```python
from build123d import *

# Parameters (mm, degrees)
BODY_DEPTH                                = 6.75
FILLET1_R                                 = 2.5
F_9_64_0_14063_DIAMETER_HOLE1_D           = 3.572002
F_9_64_0_14063_DIAMETER_HOLE1_DEPTH       = 7
F_9_64_0_14063_DIAMETER_HOLE1_CSINK_D     = 4.842002
F_9_64_0_14063_DIAMETER_HOLE1_CSINK_ANGLE = 45
F_9_64_0_14063_DIAMETER_HOLE1_TIP         = 1.073137666
MOUNT_PEG_DEPTH                           = 3
PEG_CHAMFER_SIZE                          = 0.5


with BuildPart() as part:
    # Sketch1 → body (new body)
    with BuildSketch(Plane.XY):
        with BuildLine():
            Line((6, -23.237900077), (6, -12.760161762))
            Line((6, -12.760161762), (10, -8.760161762))
            Line((10, -8.760161762), (15, -8.760161762))
            Line((15, -8.760161762), (15, -18.734993995))
            ThreePointArc((15, -18.734993995), (10.738670346, -21.463479662), (6, -23.237900077))
        make_face()
    extrude(amount=BODY_DEPTH)

    # Fillet1
    fillet1_edges = [part.edges().sort_by_distance(p)[0] for p in [
        (6, -23.237900077, 3.375),
        (6, -12.760161762, 3.375),
        (10, -8.760161762, 3.375),
        (15, -8.760161762, 3.375),
        (15, -18.734993995, 3.375),
    ]]
    fillet(fillet1_edges, radius=FILLET1_R)

    # 9/64 (0.14063) Diameter Hole1
    with Locations(Plane.ZY.offset(-6)):
        with Locations((4, -17.060161762)):
            CounterSinkHole(F_9_64_0_14063_DIAMETER_HOLE1_D / 2, F_9_64_0_14063_DIAMETER_HOLE1_CSINK_D / 2, depth=F_9_64_0_14063_DIAMETER_HOLE1_DEPTH, counter_sink_angle=F_9_64_0_14063_DIAMETER_HOLE1_CSINK_ANGLE)
            with Locations((0, 0, -(F_9_64_0_14063_DIAMETER_HOLE1_DEPTH + F_9_64_0_14063_DIAMETER_HOLE1_TIP / 2))):  # 118° drill point
                Cone(0, F_9_64_0_14063_DIAMETER_HOLE1_D / 2, F_9_64_0_14063_DIAMETER_HOLE1_TIP, mode=Mode.SUBTRACT)

    # Sketch4 → mount peg (add)
    with BuildSketch(Plane(origin=(0, 0, 0), x_dir=(-1, 0, 0), z_dir=(0, 0, -1))):
        with BuildLine():
            Line((-9.575, -19), (-9.575, -12))
            ThreePointArc((-9.575, -12), (-10.75, -10.825), (-11.925, -12))
            Line((-11.925, -12), (-11.925, -19))
            ThreePointArc((-11.925, -19), (-10.75, -20.175), (-9.575, -19))
        make_face()
    extrude(amount=MOUNT_PEG_DEPTH)

    # peg chamfer
    peg_chamfer_edges = [part.edges().sort_by_distance(p)[0] for p in [
        (11.925, -15.5, -3),
        (10.75, -10.825, -3),
        (9.575, -15.5, -3),
        (10.75, -20.175, -3),
    ]]
    chamfer(peg_chamfer_edges, length=PEG_CHAMFER_SIZE)


solid = part.part
```
Could you check a few things on this model? Use its own coordinates, in mm. A direction names the side the tool comes from. Round coordinates to 2 decimals unless told otherwise and drop trailing zeros. Write each loop counter-clockwise with the first axis right and the second up, starting at its lowest first coordinate (ties: lowest second). Pieces come first, ordered by that corner, then holes. Notation, with made-up numbers: M 25,82.25 L 72,82.25 A30 cw 72,113.25 Z; hole C -33,78.25 d2. An arc over 180 degrees is marked long. Write each question's results on one line, items separated by ' | '. Start each with the question number.
1. On a 3-axis mill with a long thin cutter (end or side, diameter ignored), from which of +Z, -Z, +X, -X, +Y, -Y can I reach the whole of each face in a straight line? I mean faces 4 (the face through (10.724, -10.825, -1.232)), 5 (the face through (11.925, -15, -1)), 6 (the face through (10.776, -20.175, -1.232)). Say none if no direction works.
2. Imagine slicing it at D-D on x = 10.75. List the corners of the cut face in (y, z) for me (3 decimals), and give its area (3 significant figures).
3. Thinking about a two-plate mould opening in Z: for faces 1 (the face through (10.066, -8.956, 3.422)), 2 (the face through (10.305, -18.645, 3.176)), 3 (the face through (11, -15, -3)), which applies, +Z half, -Z half, draft (parallel to the pull), parting line (faces both ways), or undercut?
4. Imagine slicing it at C-C on z = 1.25. List the corners of the cut face in (x, y) for me, and give its area (3 significant figures).
5. I need wall thicknesses on L1, parallel to Z at x = 14.75, y = -11.5; L2, parallel to Y at x = 10.25, z = 5.5; L3, parallel to Y at x = 9, z = 5.5. Which ranges of each line are inside material? Lowest first, please. Write a range as from..to.
6. Imagine slicing it at A-A on x = 8. List the corners of the cut face in (y, z) for me, and give its area (3 significant figures).
7. Imagine slicing it at B-B on y = -14.25. List the corners of the cut face in (x, z) for me (3 decimals).
8. I'm going to push flat-ended pins straight in: pin 1 Ø1.5 at (y, z) = (-10.5, 5) entering from -X; pin 2 Ø3 at (y, z) = (-17.06, 4) entering from -X; pin 3 Ø2 at (y, z) = (-15, -1.5) entering from +X (3 decimals). Where does each tip first touch, or does it pass through?
Result sheet:
1) face 4: -Z, +Y | face 5: -Z, +X, +Y, -Y | face 6: -Z, -Y
2) outline: M -21.458,0 L -20.175,0 L -20.175,-2.5 L -19.675,-3 L -11.325,-3 L -10.825,-2.5 L -10.825,0 L -8.777,0 L -8.777,6.75 L -21.458,6.75 Z; hole C -17.06,4 d3.572 | area: 103 mm^2
3) face 1: draft | face 2: undercut | face 3: -Z half
4) outline: M 6,-19.75 A2.5 ccw 9.49,-22.04 A24 ccw 13.95,-19.53 A2.5 ccw 15,-17.49 L 15,-11.26 A2.5 ccw 12.5,-8.76 L 11.04,-8.76 A2.5 ccw 9.27,-9.49 L 6.73,-12.03 A2.5 ccw 6,-13.8 Z | area: 101 mm^2
5) L1: z = 0..6.75 | L2: y = -21.7..-18.03, -16.09..-8.89 | L3: y = -22.2..-18.03, -16.09..-9.76
6) outline: M -22.2,0 L -10.76,0 L -10.76,6.75 L -22.2,6.75 Z; hole C -17.06,4 d3.57 | area: 67.2 mm^2
7) outline: M 6,0 L 9.575,0 L 9.575,-2.5 L 10.075,-3 L 11.425,-3 L 11.925,-2.5 L 11.925,0 L 15,0 L 15,6.75 L 6,6.75 Z
8) pin 1: stops at x = 7.51 | pin 2: stops at x = 13.17 | pin 3: stops at x = 11.925
